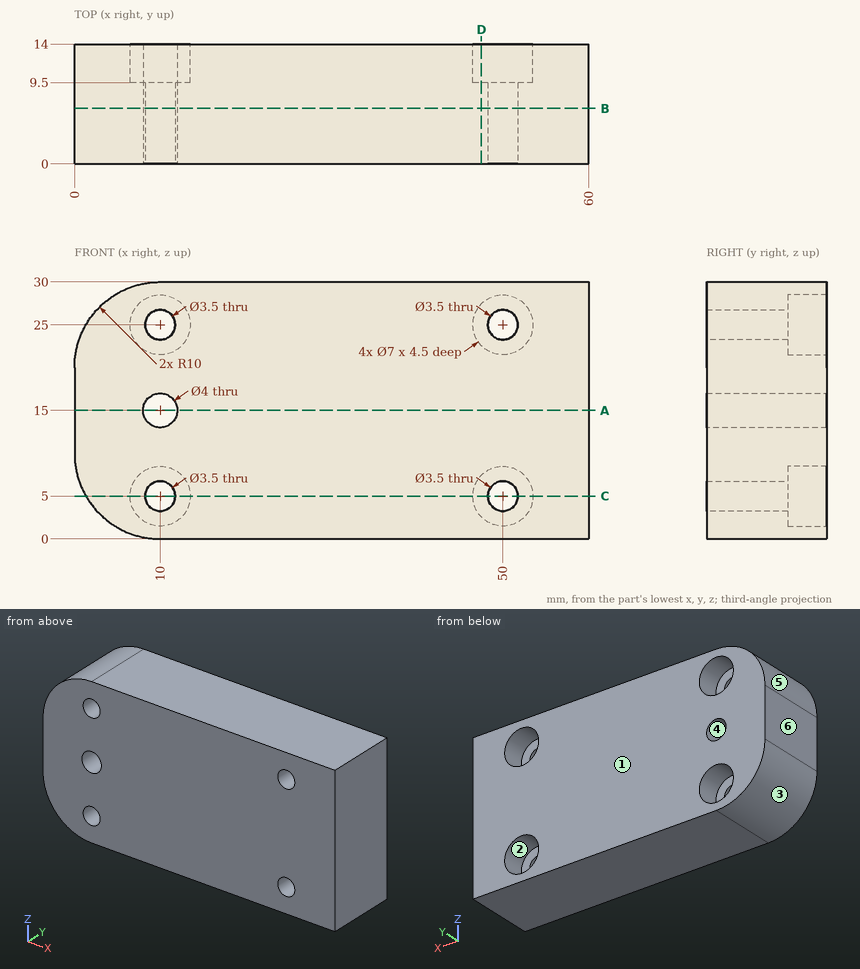
Geometry check sheet. Reference: drawing and pictorial views, mm from the part's lowest x, y, z. A direction names the side the tool comes from. Give positions to 0.01 mm unless a question says otherwise; leave off trailing zeros. Write each loop counter-clockwise with the first axis right and the second up, starting at its lowest first coordinate (ties: lowest second). Pieces come first, ordered by that corner, then holes. Notation, with made-up numbers: M -14.5,10.5 L 33.5,10.5 A19 cw 33.5,39.5 Z; hole C 62.25,44.5 d6. An arc over 180 degrees is marked long. Answer as CSV lines item,"result". Start each with the question number.
Q1. Section check A-A, the plane z = 15. Record the cut outline in (x, y), then the cut area to 3 significant figures.
Q2. Section check C-C, the plane z = 5. Record the cut outline in (x, y).
Q3. Section check B-B, the plane y = 6.5. Record the cut outline in (x, z), then the cut area to 3 significant figures.
Q4. Section check D-D, the plane x = 47.5. Record the cut outline in (y, z).
Q5. Go/stop test with flat-tipped pins: pin 1 (4 mm diameter, centred on x = 10, z = 5, fed in from +Y); pin 2 (3 mm diameter, centred on x = 50, z = 5, fed in from -Y); pin 3 (3 mm diameter, centred on y = 5, z = 5, fed in from -X). Record where each tip stops, or that it passes through.
Q6. Release check for a two-part mould opening along Z. For the marked faces 3, 4, 5 and 6 record: pulls with the +Z half, pulls with the -Z half, needs draft (parallel to the pull), parting line crosses it, or undercut.
Q7. Tool access check on the marked faces 1 and 2. Record the directions out of +Z, -Z, +X, -X, +Y, -Y that give a thin tool (end or side, any length) a straight path to the whole face; none if there is none.
Q8. Material ranges on L1, parallel to Z at x = 50, y = 5.5; L2, parallel to X at y = 12.1, z = 25; L3, parallel to X at y = 7, z = 15, recorded low to high.
Geometry says:
1,outline,"M 0,0 L 8,0 L 8,14 L 0,14 Z; M 12,0 L 60,0 L 60,14 L 12,14 Z"
1,area,"784 mm^2"
2,outline,"M 1.34,0 L 8.25,0 L 8.25,9.5 L 6.5,9.5 L 6.5,14 L 1.34,14 Z; M 11.75,0 L 48.25,0 L 48.25,9.5 L 46.5,9.5 L 46.5,14 L 13.5,14 L 13.5,9.5 L 11.75,9.5 Z; M 51.75,0 L 60,0 L 60,14 L 53.5,14 L 53.5,9.5 L 51.75,9.5 Z"
3,outline,"M 0,10 A10 ccw 10,0 L 60,0 L 60,30 L 10,30 A10 ccw 0,20 Z; hole C 10,15 d4; hole C 10,5 d3.5; hole C 10,25 d3.5; hole C 50,5 d3.5; hole C 50,25 d3.5"
3,area,"1,710 mm^2"
4,outline,"M 0,0 L 14,0 L 14,2.55 L 9.5,2.55 L 9.5,7.45 L 14,7.45 L 14,22.55 L 9.5,22.55 L 9.5,27.45 L 14,27.45 L 14,30 L 0,30 Z"
5,pin 1,"y = 9.5"
5,pin 2,"through"
5,pin 3,"x = 0.63"
6,face 3,"pulls with the -Z half"
6,face 4,"undercut"
6,face 5,"pulls with the +Z half"
6,face 6,"needs draft"
7,face 1,"+Z, -Z, +X, -X, +Y"
7,face 2,"+Y"
8,L1,"0 to 3.25, 6.75 to 23.25, 26.75 to 30"
8,L2,"1.34 to 6.5, 13.5 to 46.5, 53.5 to 60"
8,L3,"0 to 8, 12 to 60"
